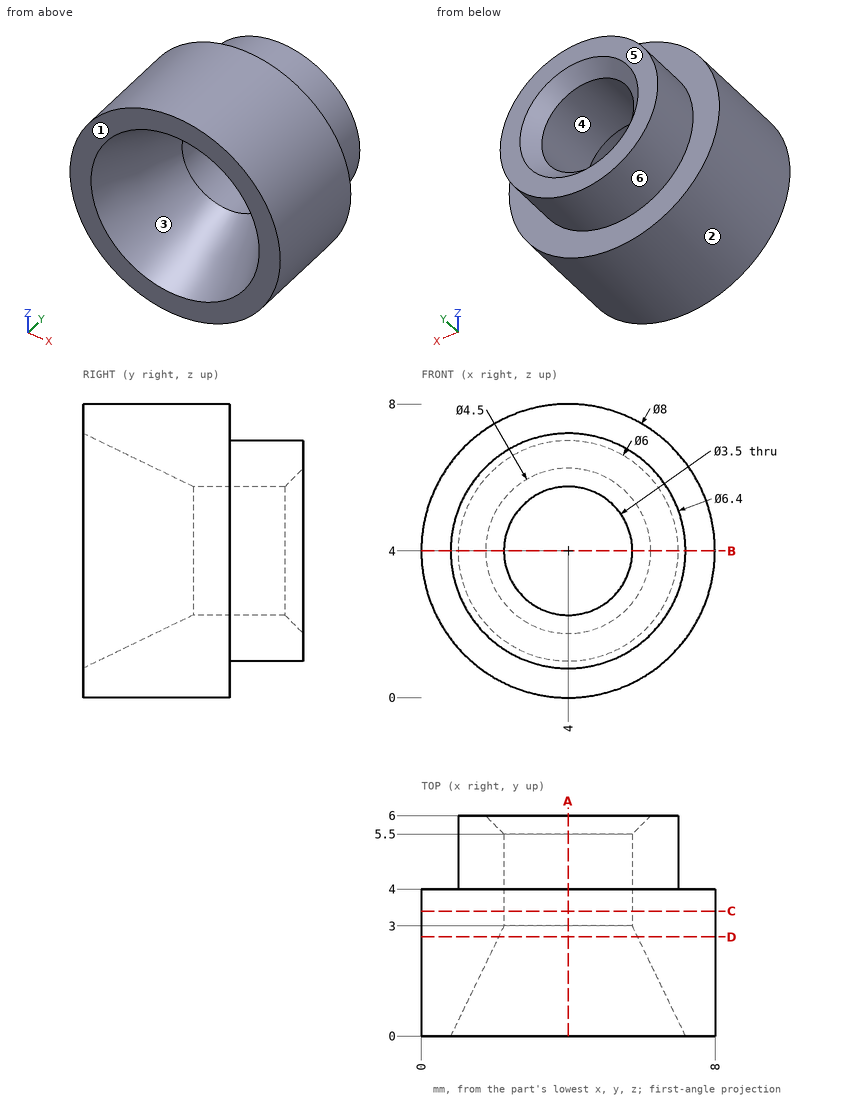
Geometry: see drawing. Coordinates: mm, zero at the bounding-box minimum. A direction names the side the tool comes from. Give positions to 0.01 mm unless a question says otherwise; leave off trailing zeros. Order: outer loops, then holes, each group sorted by start corner. A loop starts at its lowest first (then second) coordinate and runs counter-clockwise, first axis right, second up. Notation, with made-up numbers: M 63.25,52 L 85.25,52 A26 ccw 85.25,91 Z; hole C 63,30.25 d2. An arc over 180 degrees is marked long. Answer as CSV lines item,"result". Start each with the question number.
1) Line query: line 1 (Z direction, x = 4, y = 4.55); line 2 (Z direction, x = 4, y = 3.95); line 3 (Y direction, x = 6.5, z = 1.5). Output: solid intervals per line, ascending. Write a range as from..to.
2) Cut plane A-A (x = 4). Output: boundary loops of the cut face in (y, z), then the cut area to 3 significant figures.
3) Mould query, pull axis X, two halves, no side actions, for the marked faces 1, 2, 3 and 4. Classes: +X half, -X half, draft (parallel to the pull), parting line (faces both ways), or undercut.
4) First-contact query: P1, Ø3, axis at x = 4, z = 4, coming from the -Y side; P2, Ø1, axis at x = 2.5, y = 3, coming from the -Z side. Flat tips, straight axial feed; report the tip coordinate or a pass-through.
5) Cut plane C-C (y = 3.4). Output: boundary loops of the cut face in (x, z).
6) Cut plane D-D (y = 2.7). Output: boundary loops of the cut face in (x, z) (3 decimals).
7) Cut plane B-B (z = 4). Output: boundary loops of the cut face in (x, y), then the cut area to 3 significant figures.
8) Set-up query: the marked faces 5 and 6. Return all of +Z, -Z, +X, -X, +Y, -Y with unobstructed straight access to the full face (end or side cutting, diameter ignored); none if empty.
Findings below:
1,line 1,"z = 1..2.25, 5.75..7"
1,line 2,"z = 0..2.25, 5.75..8"
1,line 3,"y = 0..4"
2,outline,"M 0,0 L 4,0 L 4,1 L 6,1 L 6,1.75 L 5.5,2.25 L 3,2.25 L 0,0.8 Z; M 0,7.2 L 3,5.75 L 5.5,5.75 L 6,6.25 L 6,7 L 4,7 L 4,8 L 0,8 Z"
2,area,"18.4 mm²"
3,face 1,"draft"
3,face 2,"parting line"
3,face 3,"undercut"
3,face 4,"undercut"
4,P1,"passes through"
4,P2,"stops at z = 0.13"
5,outline,"C 4,4 d8; hole C 4,4 d3.5"
6,outline,"C 4,4 d8; hole C 4,4 d3.79"
7,outline,"M 0,0 L 0.8,0 L 2.25,3 L 2.25,5.5 L 1.75,6 L 1,6 L 1,4 L 0,4 Z; M 5.75,3 L 7.2,0 L 8,0 L 8,4 L 7,4 L 7,6 L 6.25,6 L 5.75,5.5 Z"
7,area,"18.4 mm²"
8,face 5,"+Z, -Z, +X, -X, +Y"
8,face 6,"+Y"
